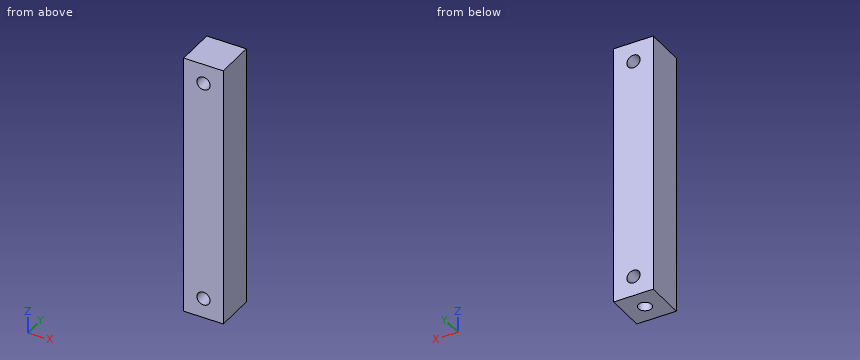
```python
from build123d import *

# Parameters (mm, degrees)
SKETCH1_W               = 60
SKETCH1_H               = 60
BOSS_EXTRUDE1_DEPTH     = 400
SKETCH2_R               = 10
CUT_EXTRUDE1_DEPTH      = 50
CUT_EXTRUDE2_DEPTH      = 60
CUT_EXTRUDE2_DEPTH_BACK = 60
SKETCH3_R               = 10
CUT_EXTRUDE3_DEPTH      = 60
CUT_EXTRUDE3_DEPTH_BACK = 60
SKETCH4_R               = 10


with BuildPart() as part:
    # Sketch1 → Boss-Extrude1 (new body)
    with BuildSketch(Plane.XY):
        Rectangle(SKETCH1_W, SKETCH1_H)
    extrude(amount=BOSS_EXTRUDE1_DEPTH)

    # Sketch2 → Cut-Extrude1 (cut)
    with BuildSketch(Plane.XY):
        Circle(SKETCH2_R)
    extrude(amount=CUT_EXTRUDE1_DEPTH, mode=Mode.SUBTRACT)

    # Sketch3 → Cut-Extrude2 (cut, two sides: drawn at the far end of the back side and taken through both)
    with BuildSketch(Plane(origin=(0, 0, 0), x_dir=(1, 0, 0), z_dir=(0, 1, 0)).offset(-CUT_EXTRUDE2_DEPTH_BACK)):
        with Locations(Location((0, -30, 0), (0, 0, 270))):
            Circle(SKETCH3_R)
    extrude(amount=CUT_EXTRUDE2_DEPTH + CUT_EXTRUDE2_DEPTH_BACK, mode=Mode.SUBTRACT)

    # Sketch4 → Cut-Extrude3 (cut, two sides: drawn at the far end of the back side and taken through both)
    with BuildSketch(Plane(origin=(0, 0, 0), x_dir=(1, 0, 0), z_dir=(0, 1, 0)).offset(-CUT_EXTRUDE3_DEPTH_BACK)):
        with Locations(Location((0, -370, 0), (0, 0, 270))):
            Circle(SKETCH4_R)
    extrude(amount=CUT_EXTRUDE3_DEPTH + CUT_EXTRUDE3_DEPTH_BACK, mode=Mode.SUBTRACT)


solid = part.part
```
The listing builds one solid part. Answer for the finished solid, in the listing's coordinates (mm). Give positions to 0.01 mm unless a question says otherwise; leave off trailing zeros. Order: outer loops, then holes, each group sorted by start corner. A loop starts at its lowest first (then second) coordinate and runs counter-clockwise, first axis right, second up. Notation, with made-up numbers: (78, -36) - (126, -36) arc R15 cw to (126, -17) - close; hole circle Ø11 at (-9, 65). An arc over 180 degrees is marked (long way). Use one line per item in the form item = value. Start each with the question number.
(1) A cutting plane is placed at C-C, the plane y = 23. Write down the section's boundary in (x, z), then the cut area to 3 significant figures.
(2) A cutting plane is placed at A-A, the plane x = 0. Write down the section's boundary in (y, z).
(3) Flat-ended cylindrical pins translate along their axes: pin 1 Ø16 at (x, z) = (0, 30) entering from +Y; pin 2 Ø6 at (x, y) = (-5, 2.5) entering from -Z. Find the tip coordinate at first contact, or state that the pin passes through.
(4) Consider line 1 (X direction, y = 7.5, z = 30); line 2 (Z direction, x = -9, y = 9.5); line 3 (Z direction, x = -6.5, y = 12.5). Determine where each line is inside the solid, lowest interval first. Write a range as from..to.
(5) A cutting plane is placed at B-B, the plane z = 370. Write down the section's boundary in (x, y), then the cut area to 3 significant figures.
Ans:
q1.outline = (-30, 0) - (30, 0) - (30, 400) - (-30, 400) - close; hole circle Ø20 at (0, 30); hole circle Ø20 at (0, 370)
q1.area = 23,400 mm^2
q2.outline = (-30, 0) - (-10, 0) - (-10, 20) - (-30, 20) - close; (-30, 40) - (-10, 40) - (-10, 50) - (10, 50) - (10, 40) - (30, 40) - (30, 360) - (-30, 360) - close; (-30, 380) - (30, 380) - (30, 400) - (-30, 400) - close; (10, 0) - (30, 0) - (30, 20) - (10, 20) - close
q3.pin_1 = through
q3.pin_2 = 50
q4.line_1 = -30..-10, 10..30
q4.line_2 = 0..25.64, 34.36..365.64, 374.36..400
q4.line_3 = 0..22.4, 37.6..362.4, 377.6..400
q5.outline = (-30, -30) - (-10, -30) - (-10, 30) - (-30, 30) - close; (10, -30) - (30, -30) - (30, 30) - (10, 30) - close
q5.area = 2,400 mm^2
